Here's how the part is built. I have some questions about the finished solid (model axes, mm). Face numbers are marked on the shaded views. Coordinates: 2 decimals unless noted, no trailing zeros. Order: outer loops, then holes, each group sorted by start corner. A loop starts at its lowest first (then second) coordinate and runs counter-clockwise, first axis right, second up. Notation, with made-up numbers: (62.25, 50.5) -> (76.25, 50.5) arc R9 cw to (76.25, 63.5) -> close; hole circle Ø2 at (37.25, -19.5). An arc over 180 degrees is marked (long way). One line per item, written item: value. Start each with the question number.
```python
from build123d import *

# Parameters (mm, degrees)
SKETCH1_R               = 49.53
SKETCH1_R_2             = 38.1
BOSS_EXTRUDE1_DEPTH     = 12.7
CUT_EXTRUDE1_DEPTH      = 72.188003203
CUT_EXTRUDE1_DEPTH_BACK = 72.188003203
SKETCH8_W               = 6.35
SKETCH8_H               = 75.934955718
CUT_EXTRUDE3_DEPTH      = 71.893836562
SKETCH9_W               = 6.35
SKETCH9_H               = 12.7
CUT_EXTRUDE4_DEPTH      = 2.54
SKETCH10_R              = 1.6
CUT_EXTRUDE5_DEPTH      = 5.08


with BuildPart() as part:
    # Sketch1 → Boss-Extrude1 (new body)
    # profile 1 of 2: a face of its own
    with BuildSketch(Plane(origin=(0, 0, 0), x_dir=(1, 0, 0), z_dir=(0, 1, 0))):
        with Locations(Location((0, 0, 0), (0, 0, 270))):
            Circle(SKETCH1_R)
        Circle(SKETCH1_R_2, mode=Mode.SUBTRACT)
    # profile 2 of 2: a face of its own
    with BuildSketch(Plane(origin=(0, 0, 0), x_dir=(1, 0, 0), z_dir=(0, 1, 0))):
        with BuildLine():
            Line((-3.175, 37.967477859), (-3.175, -37.967477859))
            ThreePointArc((-3.175, -37.967477859), (0, -38.1), (3.175, -37.967477859))
            Line((3.175, -37.967477859), (3.175, 37.967477859))
            ThreePointArc((3.175, 37.967477859), (0, 38.1), (-3.175, 37.967477859))
        make_face()
    extrude(amount=BOSS_EXTRUDE1_DEPTH)

    # Sketch7 → Cut-Extrude1 (cut, two sides: drawn at the far end of the back side and taken through both)
    with BuildSketch(Plane.XZ.offset(-CUT_EXTRUDE1_DEPTH_BACK)):
        with BuildLine():
            Line((-49.106263984, -6.464962301), (-37.774049218, -4.973047924))
            ThreePointArc((-37.774049218, -4.973047924), (-38.1, 0), (-37.774049218, 4.973047924))
            Line((-37.774049218, 4.973047924), (-49.106263984, 6.464962301))
            ThreePointArc((-49.106263984, 6.464962301), (-49.53, 0), (-49.106263984, -6.464962301))
        make_face()
        with BuildLine():
            Line((49.106263984, 6.464962301), (37.774049218, 4.973047924))
            ThreePointArc((37.774049218, 4.973047924), (38.1, 0), (37.774049218, -4.973047924))
            Line((37.774049218, -4.973047924), (49.106263984, -6.464962301))
            ThreePointArc((49.106263984, -6.464962301), (49.53, 0), (49.106263984, 6.464962301))
        make_face()
    extrude(amount=CUT_EXTRUDE1_DEPTH + CUT_EXTRUDE1_DEPTH_BACK, mode=Mode.SUBTRACT)

    # Sketch8 → Cut-Extrude3 (cut, through all)
    with BuildSketch(Plane(origin=(0, 12.7, 0), x_dir=(1, 0, 0), z_dir=(0, 1, 0))):
        Rectangle(SKETCH8_W, SKETCH8_H)
    extrude(amount=-CUT_EXTRUDE3_DEPTH, mode=Mode.SUBTRACT)


with BuildPart() as body_2:
    # of the pieces the cut leaves, the one that is kept (cut_extrude3_keep)
    add(part.part.solids().sort_by_distance((-49.106263984, 0, 6.464962301))[0])

    # Sketch9 → Cut-Extrude4 (cut)
    with BuildSketch(Plane(origin=(0, 0, 37.967477859), x_dir=(-1, 0, 0), z_dir=(0, 0, -1))):
        with Locations((0, 6.35)):
            Rectangle(SKETCH9_W, SKETCH9_H)
    extrude(amount=-CUT_EXTRUDE4_DEPTH, mode=Mode.SUBTRACT)

    # Sketch10 → Cut-Extrude5 (cut)
    with BuildSketch(Plane(origin=(0, 12.7, 0), x_dir=(1, 0, 0), z_dir=(0, 1, 0))):
        with Locations(Location((0, -44.885010743, 0), (0, 0, 270))):
            Circle(SKETCH10_R)
    extrude(amount=-CUT_EXTRUDE5_DEPTH, mode=Mode.SUBTRACT)


solid = body_2.part
```
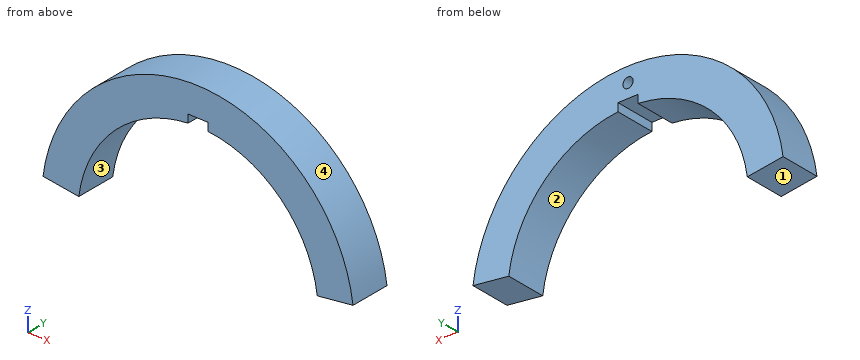
Q1. I need wall thicknesses on line 1 (X direction, y = 4, z = 8); line 2 (Z direction, x = 0.5, y = 6.75); line 3 (X direction, y = 3.75, z = 30). Which ranges of each line are inside material? Lowest first, please.
Q2. Imagine slicing it at A-A (z = 28). Write out the boundary of the cut face in (x, y).
Q3. For P1, Ø1.3, axis at y = 8.5, z = 39, coming from the +X side; P2, Ø1.6, axis at x = 0, z = 45.5, coming from the +Y side; P3, Ø0.8, axis at y = 9.5, z = 39.5, coming from the -X side, each with a flat end and sliding along its axis, tell me the tip position at first contact or that it passes through.
Q4. If we mould it in two halves opening along X, with no side actions, what happens to the marked faces 1, 2, 3 and 4? For each: +X half, -X half, draft (parallel to the pull), parting line (faces both ways), or undercut.
Q5. Imagine slicing it at C-C (x = 0). Write out the boundary of the cut face in (y, z).
Q6. Imagine slicing it at D-D (y = 3.5). Write out the boundary of the cut face in (x, z) (3 decimals), plus the area to 3 significant figures.
Q7. Imagine slicing it at B-B (y = 11.75). Write out the boundary of the cut face in (x, z) (3 decimals), plus the area to 3 significant figures.
Completed:
1. line 1: x = -48.88 to -37.25, 37.25 to 48.88
1. line 2: z = 40.51 to 49.53
1. line 3: x = -39.41 to -23.49, 23.49 to 39.41
2. outline: (-40.86, 0) -> (-25.84, 0) -> (-25.84, 12.7) -> (-40.86, 12.7) -> close; (25.84, 0) -> (40.86, 0) -> (40.86, 12.7) -> (25.84, 12.7) -> close
3. P1: stops at x = 31.34
3. P2: stops at y = 7.62
3. P3: stops at x = -30.4
4. face 1: -X half
4. face 2: undercut
4. face 3: undercut
4. face 4: parting line
5. outline: (0, 40.51) -> (12.7, 40.51) -> (12.7, 43.29) -> (7.62, 43.29) -> (7.62, 46.49) -> (12.7, 46.49) -> (12.7, 49.53) -> (0, 49.53) -> close
6. outline: (-49.106, 6.465) -> (-37.774, 4.973) arc R38.1 cw to (-3.175, 37.967) -> (-3.175, 40.507) -> (3.175, 40.507) -> (3.175, 37.967) arc R38.1 cw to (37.774, 4.973) -> (49.106, 6.465) arc R49.53 ccw to start
6. area: 1,430 mm2
7. outline: (-49.106, 6.465) -> (-37.774, 4.973) arc R38.1 cw to (-3.175, 37.967) -> (-3.175, 40.507) -> (3.175, 40.507) -> (3.175, 37.967) arc R38.1 cw to (37.774, 4.973) -> (49.106, 6.465) arc R49.53 ccw to start; hole circle Ø3.2 at (0, 44.885)
7. area: 1,420 mm2
